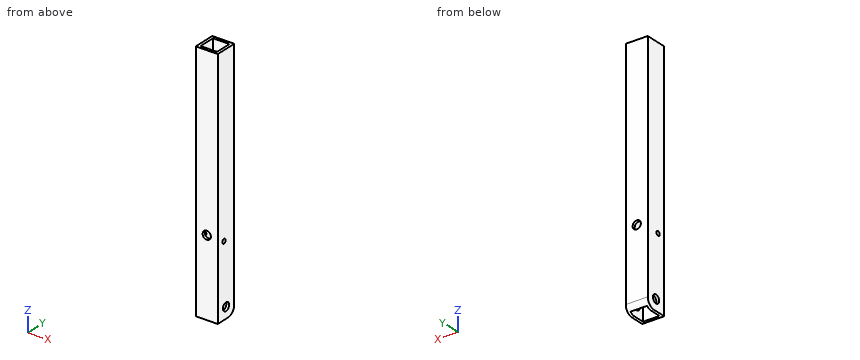
Autodesk Inventor part; units mm, degrees
ref_plane "YZ Plane" through (0, 0, 0) normal (1, 0, 0) x (0, 1, 0)
ref_plane "XZ Plane" through (0, 0, 0) normal (0, 1, 0) x (-1, 0, 0)
ref_plane "XY Plane" through (0, 0, 0) normal (0, 0, 1) x (1, 0, 0)
sketch "Sketch1" plane through (0, 0, 0) normal (0, 0, 1) x (1, 0, 0)
  line L0 (-12.7, -12.7) -> (12.7, -12.7)
  line L1 (12.7, -12.7) -> (12.7, 12.7)
  line L2 (12.7, 12.7) -> (-12.7, 12.7)
  line L3 (-12.7, 12.7) -> (-12.7, -12.7)
  line L4 (-12.7, -12.7) -> (12.7, 12.7) construction
  line L5 (12.7, -12.7) -> (-12.7, 12.7) construction
  line L6 (-9.525, -9.525) -> (9.525, -9.525)
  line L7 (9.525, -9.525) -> (9.525, 9.525)
  line L8 (9.525, 9.525) -> (-9.525, 9.525)
  line L9 (-9.525, 9.525) -> (-9.525, -9.525)
  line L10 (-9.525, -9.525) -> (9.525, 9.525) construction
  line L11 (9.525, -9.525) -> (-9.525, 9.525) construction
  point P0 (0, 0)
  dimension "d0" = 25.4
  dimension "d1" = 3.175
extrude "Extrusion1" add sketch "Sketch1" along normal mid plane 282.575
sketch "Sketch2" plane through (12.7, -12.7, 141.2875) normal (1, 0, 0) x (0, 0, -1)
  line L0 (0, 22.225) -> (0, 3.175) construction
  line L1 (0, 12.7) -> (282.575, 12.7) construction
  line L2 (282.575, 3.175) -> (282.575, 22.225) construction
  circle A0 centre (269.875, 12.7) radius 4.7625
  circle A1 centre (200.025, 9.525) radius 2.54
  point P0 (141.2875, 12.7)
  dimension "d4" = 9.525
  dimension "d5" = 12.7
  dimension "d19" = 5.08
  dimension "d20" = 69.85
  dimension "d21" = 3.175
extrude "Extrusion2" cut sketch "Sketch2" against normal through all
sketch "Sketch3" plane through (-12.7, 12.7, 141.2875) normal (0, 1, 0) x (1, 0, 0)
  line L0 (0, 0) -> (25.4, 0) construction
  line L1 (22.225, 282.575) -> (3.175, 282.575) construction
  line L2 (0, 282.575) -> (0, 0)
  line L3 (3.175, 282.575) -> (22.225, 282.575) construction
  line L4 (3.175, 282.575) -> (3.175, 0) construction
  circle A0 centre (12.7, 193.675) radius 4.7625
  line L5 (25.4, 282.575) -> (25.4, 0)
  point P0 (12.7, 141.2875)
  dimension "d15" = 3.175
  dimension "d22" = 88.9
  dimension "d23" = 12.7
  dimension "d24" = 9.525
extrude "Extrusion3" cut sketch "Sketch3" against normal through all
fillet "Fillet1" radius 9.525 1 edges at (0, 12.7, -141.2875)
properties part number "pivot arm" material "Aluminum 6061"
Geometry check sheet. Reference: the model listing, model coordinates, mm. Give positions to 0.01 mm unless a question says otherwise; leave off trailing zeros. Loops run counter-clockwise (first coordinate to the right, second up) from the corner with the lowest first, then second, coordinate; pieces in that order, holes last. Notation, with made-up numbers: M 66.5,31 L 84.5,31 A15 ccw 84.5,43 Z; hole C 11.25,42 d10. An arc over 180 degrees is marked long. Write each question's results on one line, items separated by ' | '.
1) Section check A-A, the plane x = 0. Count the separate pieces of the cut face and the enclosed holes in it, plus the area to 3 significant figures.
Answers follow:
separate pieces: 4 | enclosed holes: 0 | area: 1,720 mm2
2) Gauge pin test, flat end, axial feed: pin 1 (8 mm diameter, centred on x = 9, y = -4.5, fed in from -Z). Record the tip position at first contact, or that the pin passes through.
Answers follow:
pin 1: z = -141.29
3) Thickness scan on line 1 (Y direction, x = -7, z = 82.5) (3 decimals); line 2 (Z direction, x = -10, y = 2.25). Record the ranges inside material, lowest first.
Answers follow:
line 1: -12.7 to -9.525, 9.525 to 12.7 | line 2: -141.29 to -132.78, -124.39 to 141.29
4) Section check B-B, the plane z = 65. Record the boundary of the cut face in (x, y) (3 decimals), plus the area to 3 significant figures.
Answers follow:
outline: M -12.7,-12.7 L 12.7,-12.7 L 12.7,12.7 L -12.7,12.7 Z; hole M -9.525,-9.525 L 9.525,-9.525 L 9.525,9.525 L -9.525,9.525 Z | area: 282 mm2
